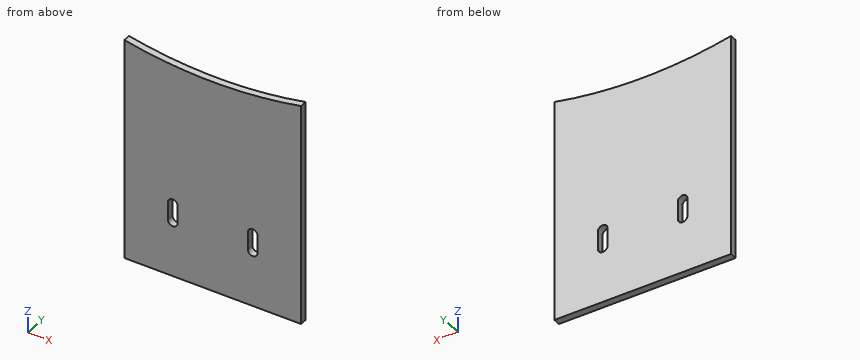
from build123d import *

# Parameters (mm, degrees)
SM_BASE_FLANGE_1_DEPTH = 16


# Sheet-metal steps are written as plain solids
with BuildPart() as part:
    # Sketch 1 → 基体-法兰1 (new body)
    with BuildSketch(Plane(origin=(0, 0, 0), x_dir=(1, 0, 0), z_dir=(0, 1, 0))):
        with BuildLine():
            Line((-200, 964.992357483), (-200, 1467.5))
            Line((-200, 1467.5), (200, 1467.5))
            Line((200, 1467.5), (200, 964.992357483))
            ThreePointArc((200, 964.992357483), (0, 985.5), (-200, 964.992357483))
        make_face()
        with BuildLine():
            Line((-79.5, 1341.5), (-79.5, 1301.5))
            ThreePointArc((-79.5, 1301.5), (-90.5, 1290.5), (-101.5, 1301.5))
            Line((-101.5, 1301.5), (-101.5, 1341.5))
            ThreePointArc((-101.5, 1341.5), (-90.5, 1352.5), (-79.5, 1341.5))
        make_face(mode=Mode.SUBTRACT)
        with BuildLine():
            Line((79.5, 1301.5), (79.5, 1341.5))
            ThreePointArc((79.5, 1341.5), (90.5, 1352.5), (101.5, 1341.5))
            Line((101.5, 1341.5), (101.5, 1301.5))
            ThreePointArc((101.5, 1301.5), (90.5, 1290.5), (79.5, 1301.5))
        make_face(mode=Mode.SUBTRACT)
    extrude(amount=SM_BASE_FLANGE_1_DEPTH)


solid = part.part
Work out the finished part from the listing and answer in its coordinate system (mm). Give positions to 0.01 mm unless a question says otherwise; leave off trailing zeros. Order: outer loops, then holes, each group sorted by start corner. A loop starts at its lowest first (then second) coordinate and runs counter-clockwise, first axis right, second up. Notation, with made-up numbers: (9.5, 53.5) - (57.5, 53.5) arc R22 ccw to (57.5, 89.5) - close; hole circle Ø5 at (-33.5, 48.5). An arc over 180 degrees is marked (long way). Answer as CSV lines item,"result". Start each with the question number.
Q1. The part is cut by section A-A (y = 6). Write down the section's boundary in (x, z), then the cut area to 3 significant figures.
Q2. Find the intervals of material crossed by L1, parallel to X at y = 12.5, z = -1337.5; L2, parallel to X at y = 8.5, z = -1295; L3, parallel to Z at x = -86, y = 4.75, in increasing order. Write a range as [from, to].
Q3. The part is cut by section D-D (x = 19). Write down the section's boundary in (y, z).
Q4. The part is cut by section C-C (x = -29.5). Write down the section's boundary in (y, z), then the cut area to 3 significant figures.
Q5. The part is cut by section B-B (x = 90.5). Write down the section's boundary in (y, z), then the cut area to 3 significant figures.
Check result:
1,outline,"(-200, -1467.5) - (200, -1467.5) - (200, -964.99) arc R985.5 cw to (-200, -964.99) - close; hole (-101.5, -1341.5) arc R11 ccw to (-79.5, -1341.5) - (-79.5, -1301.5) arc R11 ccw to (-101.5, -1301.5) - close; hole (79.5, -1341.5) arc R11 ccw to (101.5, -1341.5) - (101.5, -1301.5) arc R11 ccw to (79.5, -1301.5) - close"
1,area,"193,000 mm²"
2,L1,"x = [-200, -101.5], [-79.5, 79.5], [101.5, 200]"
2,L2,"x = [-200, -99.37], [-81.63, 81.63], [99.37, 200]"
2,L3,"z = [-1467.5, -1351.54], [-1291.46, -981.74]"
3,outline,"(0, -1467.5) - (16, -1467.5) - (16, -985.32) - (0, -985.32) - close"
4,outline,"(0, -1467.5) - (16, -1467.5) - (16, -985.06) - (0, -985.06) - close"
4,area,"7,720 mm²"
5,outline,"(0, -1467.5) - (16, -1467.5) - (16, -1352.5) - (0, -1352.5) - close; (0, -1290.5) - (16, -1290.5) - (16, -981.34) - (0, -981.34) - close"
5,area,"6,790 mm²"
